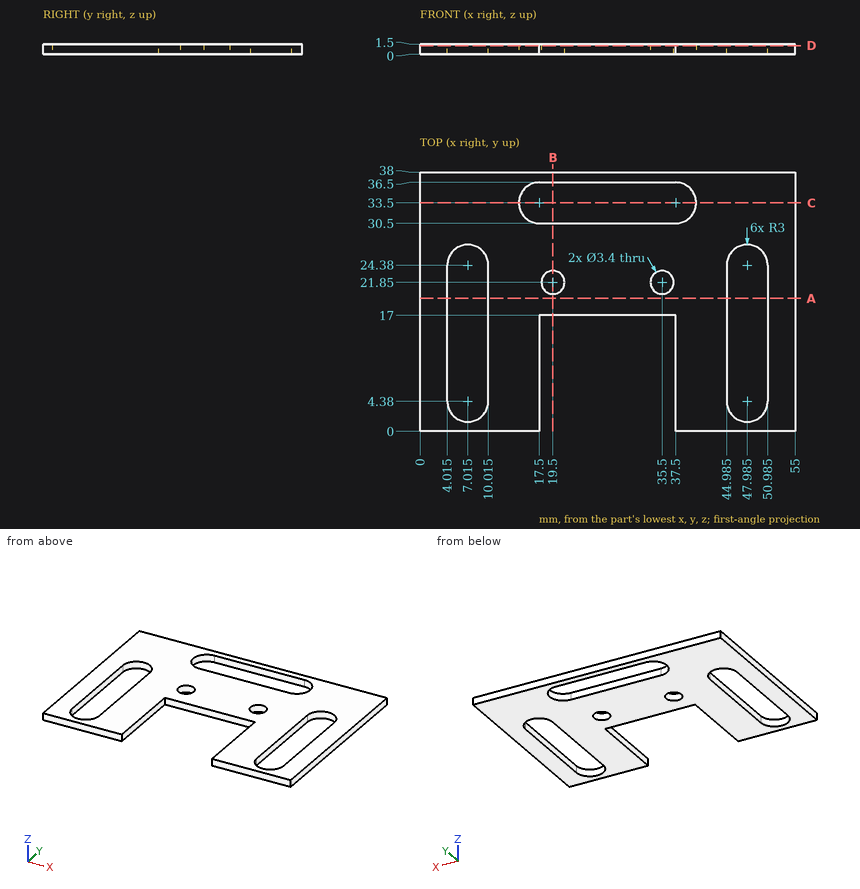
The drawing under review shows one solid part. Ordinate dimensions are in mm from its lowest x, y, z. Round coordinates to 2 decimals unless told otherwise and drop trailing zeros. Loops run counter-clockwise (first coordinate to the right, second up) from the corner with the lowest first, then second, coordinate; pieces in that order, holes last. Notation, with made-up numbers: (26, -34) - (32, -34) arc R24 cw to (32, -12) - close; hole circle Ø1 at (6.25, 52). An arc over 180 degrees is marked (long way). One line per question, with ' | ' between items.
Q1. For line 1 along X through (y, z) = (6.5, 0.75) (3 decimals); line 2 along Y through (x, z) = (19.5, 0.9); line 3 along X through (y, z) = (20, 0.8) (3 decimals), list the stretches that pass through material, from the lowest coordinate up. Write a range as [from, to].
Taken from the geometry:
line 1: x = [0, 4.015], [10.015, 17.5], [37.5, 44.985], [50.985, 55] | line 2: y = [17, 20.15], [23.55, 30.5], [36.5, 38] | line 3: x = [0, 4.015], [10.015, 44.985], [50.985, 55]
Q2. Take a section at D-D (z = 1.25). Give the boundary of the cut face in (x, y) (3 decimals), and give its area (3 significant figures).
Taken from the geometry:
outline: (0, 0) - (17.5, 0) - (17.5, 17) - (37.5, 17) - (37.5, 0) - (55, 0) - (55, 38) - (0, 38) - close; hole (4.015, 4.38) arc R3 ccw to (10.015, 4.38) - (10.015, 24.38) arc R3 ccw to (4.015, 24.38) - close; hole (17.5, 30.5) - (37.5, 30.5) arc R3 ccw to (37.5, 36.5) - (17.5, 36.5) arc R3 ccw to start; hole circle Ø3.4 at (19.5, 21.85); hole circle Ø3.4 at (35.5, 21.85); hole (44.985, 4.38) arc R3 ccw to (50.985, 4.38) - (50.985, 24.38) arc R3 ccw to (44.985, 24.38) - close | area: 1,290 mm²
Q3. Take a section at C-C (y = 33.5). Give the boundary of the cut face in (x, z), and give its area (3 significant figures).
Taken from the geometry:
outline: (0, 0) - (14.5, 0) - (14.5, 1.5) - (0, 1.5) - close; (40.5, 0) - (55, 0) - (55, 1.5) - (40.5, 1.5) - close | area: 43.5 mm²
Q4. Take a section at B-B (x = 19.5). Give the boundary of the cut face in (y, z), and give its area (3 significant figures).
Taken from the geometry:
outline: (17, 0) - (20.15, 0) - (20.15, 1.5) - (17, 1.5) - close; (23.55, 0) - (30.5, 0) - (30.5, 1.5) - (23.55, 1.5) - close; (36.5, 0) - (38, 0) - (38, 1.5) - (36.5, 1.5) - close | area: 17.4 mm²
Q5. Take a section at A-A (y = 19.5). Give the boundary of the cut face in (x, z) (3 decimals), and give its area (3 significant figures).
Taken from the geometry:
outline: (0, 0) - (4.015, 0) - (4.015, 1.5) - (0, 1.5) - close; (10.015, 0) - (44.985, 0) - (44.985, 1.5) - (10.015, 1.5) - close; (50.985, 0) - (55, 0) - (55, 1.5) - (50.985, 1.5) - close | area: 64.5 mm²
